```python
from build123d import *

# Parameters (mm, degrees)
F0_W           = 13.375
F0_H           = 2
F1_DEPTH       = 25
F2_R           = 1.75
F3_DEPTH       = 2
F4_W           = 11.3
F4_H           = 33
F5_DEPTH       = 25
F5_DEPTH_BACK  = 11.5
F6_W           = 26
F6_H           = 6.5
F7_DEPTH       = 33
F9_DEPTH       = 33
F11_DEPTH      = 19.75
F11_DEPTH_BACK = 6.25
F12_R          = 1.375
F13_DEPTH      = 4.8
F14_W          = 5.5
F14_H          = 5.5
F15_DEPTH      = 1.5
F16_T1_DEPTH   = 27.75
F16_T3_DEPTH   = 27.75
F16_T5_DEPTH   = 59
F17_T1_DEPTH   = 59.021567647
F17_T3_DEPTH   = 59.021567647
F18_T1_DEPTH   = 6.4746360003
F18_T3_DEPTH   = 20.7323463904
F18_T5_DEPTH   = 52.0573463904
F18_T7_DEPTH   = 15.4323463904
F18_T9_DEPTH   = 14.5286731952
F18_T11_DEPTH  = 6.3286731952
F18_T13_DEPTH  = 6.4746360003
F18_T15_DEPTH  = 1.5286731952
F18_T17_DEPTH  = 7.7786731952
F18_T19_DEPTH  = 7.7786731952
F18_T24_DEPTH  = 4.8857735151
F18_T29_DEPTH  = 10.5573463904
F18_T35_DEPTH  = 4.8857735151
F18_T45_DEPTH  = 14.5286731952
F18_T49_DEPTH  = 7.3573463904
F18_T56_DEPTH  = 8.8073463904
F18_T60_DEPTH  = 2.5573463904
F18_T67_DEPTH  = 4.8857735151
F18_T71_DEPTH  = 10.5573463904
F18_T78_DEPTH  = 10.5573463904
F18_T82_DEPTH  = 4.8857735151
F18_T89_DEPTH  = 2.5573463904
F18_T93_DEPTH  = 8.8073463904


# Not quite as in the source:
# - a fillet or chamfer that OpenCascade refuses, or shapes differently, is made with other operations: its cross-section is extruded or revolved along the edge and cut away or added


with BuildPart() as f1:
    # F0 (on Right) → F1 (new body, symmetric)
    with BuildSketch(Plane.YZ):
        with Locations((6.6875, 1)):
            Rectangle(F0_W, F0_H)
    extrude(amount=F1_DEPTH, both=True)

    # F2 (on face) → F3 (cut, through all)
    with BuildSketch(Plane.XY.offset(2)):
        with Locations((-13, 4)):
            Circle(F2_R)
        with Locations((13, 4)):
            Circle(F2_R)
    extrude(amount=-F3_DEPTH, mode=Mode.SUBTRACT)

    # F4 (on Right) → F5 (join, two sides)
    with BuildSketch(Plane.YZ) as f5_sk:
        with Locations((-5.65, -14.5)):
            Rectangle(F4_W, F4_H)
    extrude(amount=F5_DEPTH)
    extrude(f5_sk.sketch, amount=-F5_DEPTH_BACK)

    # F6 (on face) → F7 (cut, through all)
    with BuildSketch(Plane(origin=(0, 0, -31), x_dir=(1, 0, 0), z_dir=(0, 0, -1))):
        with Locations((6.75, 8.05)):
            Rectangle(F6_W, F6_H)
    extrude(amount=-F7_DEPTH, mode=Mode.SUBTRACT)

    # F8 (on face) → F9 (cut, through all)
    with BuildSketch(Plane(origin=(0, 0, -31), x_dir=(1, 0, 0), z_dir=(0, 0, -1))):
        Polygon((13, 4.8), (0.5, 4.8), (2.5, 2.8), (11, 2.8), align=None)
    extrude(amount=-F9_DEPTH, mode=Mode.SUBTRACT)

    # F10 (on Right) → F11 (cut, two sides)
    with BuildSketch(Plane.YZ) as f11_sk:
        Polygon((-4.8, -31), (-2.8, -31), (-4.8, -19), align=None)
    extrude(amount=F11_DEPTH, mode=Mode.SUBTRACT)
    extrude(f11_sk.sketch, amount=-F11_DEPTH_BACK, mode=Mode.SUBTRACT)

    # F12 (on face) → F13 (cut, through all)
    with BuildSketch(Plane.XZ.offset(4.8)):
        with Locations((-2.5, -16)):
            Circle(F12_R)
        with Locations((16, -16)):
            Circle(F12_R)
    extrude(amount=-F13_DEPTH, mode=Mode.SUBTRACT)

    # F14 (on face) → F15 (cut)
    with BuildSketch(Plane(origin=(0, 0, 0), x_dir=(-1, 0, 0), z_dir=(0, 1, 0))):
        with Locations((-16, -16)):
            Rectangle(F14_W, F14_H)
        with Locations((2.5, -16)):
            Rectangle(F14_W, F14_H)
    extrude(amount=-F15_DEPTH, mode=Mode.SUBTRACT)

    # F16: fillet of radius 4.5 on 3 edges, made by hand

    # F16_s2 → F16_t1 (cut)
    with BuildSketch(Plane.YZ.offset(-22.75)):
        with BuildLine():
            ThreePointArc((-11.3, -26.5), (-9.9819805153, -29.6819805153), (-6.8, -31))
            Line((-6.8, -31), (-11.3, -31))
            Line((-11.3, -31), (-11.3, -26.5))
        make_face()
    extrude(amount=F16_T1_DEPTH, mode=Mode.SUBTRACT)

    # F16_s4 → F16_t3 (cut)
    with BuildSketch(Plane.YZ.offset(8.5)):
        with BuildLine():
            ThreePointArc((-11.3, -26.5), (-9.9819805153, -29.6819805153), (-6.8, -31))
            Line((-6.8, -31), (-11.3, -31))
            Line((-11.3, -31), (-11.3, -26.5))
        make_face()
    extrude(amount=F16_T3_DEPTH, mode=Mode.SUBTRACT)

    # F16_s6 → F16_t5 (cut)
    with BuildSketch(Plane.YZ.offset(-22.75)):
        with BuildLine():
            ThreePointArc((0, -26.5), (-1.3180194847, -29.6819805153), (-4.5, -31))
            Line((-4.5, -31), (0, -31))
            Line((0, -31), (0, -26.5))
        make_face()
    extrude(amount=F16_T5_DEPTH, mode=Mode.SUBTRACT)

    # F17: chamfer of 6 x 10.3923048454 on 2 edges, made by hand

    # F17_s2 → F17_t1 (cut)
    with BuildSketch(Plane.YZ.offset(-38.3857838235)):
        Polygon((-5.3, 2), (-11.3, -8.3923048454), (-11.3, 2), align=None)
    extrude(amount=F17_T1_DEPTH, mode=Mode.SUBTRACT)

    # F17_s4 → F17_t3 (cut)
    with BuildSketch(Plane.YZ.offset(-7.1357838235)):
        Polygon((-5.3, 2), (-11.3, -8.3923048454), (-11.3, 2), align=None)
    extrude(amount=F17_T3_DEPTH, mode=Mode.SUBTRACT)

    # F18: chamfer of 0.4 on 16 edges, made by hand

    # F18_s2 → F18_t1 (cut)
    with BuildSketch(Plane.YZ.offset(19.1376819998)):
        Polygon((-5.4154700538, 1.8), (-5.0690598923, 2), (-5.3, 2), align=None)
    extrude(amount=F18_T1_DEPTH, mode=Mode.SUBTRACT)

    # F18_s4 → F18_t3 (cut)
    with BuildSketch(Plane.XZ.offset(-14.4036731952)):
        Polygon((25, 1.6), (24.6, 2), (25, 2), align=None)
    extrude(amount=F18_T3_DEPTH, mode=Mode.SUBTRACT)

    # F18_s6 → F18_t5 (cut)
    with BuildSketch(Plane.YZ.offset(-26.0286731952)):
        Polygon((13.375, 1.6), (12.975, 2), (13.375, 2), align=None)
    extrude(amount=F18_T5_DEPTH, mode=Mode.SUBTRACT)

    # F18_s8 → F18_t7 (cut)
    with BuildSketch(Plane.XZ.offset(-14.4036731952)):
        Polygon((-25, 1.6), (-24.6, 2), (-25, 2), align=None)
    extrude(amount=F18_T7_DEPTH, mode=Mode.SUBTRACT)

    # F18_s10 → F18_t9 (cut)
    with BuildSketch(Plane.YZ.offset(-26.0286731952)):
        Polygon((0, 1.6), (0.4, 2), (0, 2), align=None)
    extrude(amount=F18_T9_DEPTH, mode=Mode.SUBTRACT)

    # F18_s12 → F18_t11 (cut)
    with BuildSketch(Plane.XZ):
        Polygon((-11.5, 1.6), (-11.1, 2), (-11.5, 2), align=None)
    extrude(amount=F18_T11_DEPTH, mode=Mode.SUBTRACT)

    # F18_s14 → F18_t13 (cut)
    with BuildSketch(Plane.YZ.offset(-12.1123180002)):
        Polygon((-5.4154700538, 1.8), (-5.0690598923, 2), (-5.3, 2), align=None)
    extrude(amount=F18_T13_DEPTH, mode=Mode.SUBTRACT)

    # F18_s16 → F18_t15 (cut)
    with BuildSketch(Plane.XZ.offset(4.8)):
        Polygon((-6.25, 1.6), (-6.65, 2), (-6.25, 2), align=None)
        Polygon((19.75, 1.6), (20.15, 2), (19.75, 2), align=None)
    extrude(amount=F18_T15_DEPTH, mode=Mode.SUBTRACT)

    # F18_s18 → F18_t17 (cut)
    with BuildSketch(Plane.YZ.offset(-6.25)):
        Polygon((-4.8, 1.6), (-4.4, 2), (-4.8, 2), align=None)
    extrude(amount=F18_T17_DEPTH, mode=Mode.SUBTRACT)

    # F18_s20 → F18_t19 (cut)
    with BuildSketch(Plane.YZ.offset(11.9713268048)):
        Polygon((-4.8, 1.6), (-4.4, 2), (-4.8, 2), align=None)
    extrude(amount=F18_T19_DEPTH, mode=Mode.SUBTRACT)


with BuildPart() as f18_tool22:
    # F18_s23 → F18_t24 (new body)
    with BuildSketch(Plane(origin=(-2.8773817919, -2.8773817919, 0), x_dir=(0, 0, 1), z_dir=(0.7071067812, 0.7071067812, 0))):
        Polygon((1.6, 3.7476659403), (2, 3.3476659403), (2, 3.7476659403), align=None)
    extrude(amount=F18_T24_DEPTH)

    split(bisect_by=Plane.XZ.offset(2.8), keep=Keep.TOP)


with BuildPart() as f1_1:
    add(f1.part)

    # F18_t21: cut F18_tool22
    add(f18_tool22.part, mode=Mode.SUBTRACT)


with BuildPart() as f18_tool27:
    # F18_s28 → F18_t29 (new body)
    with BuildSketch(Plane.YZ.offset(1.4713268048)):
        Polygon((-2.8, 1.6), (-2.4, 2), (-2.8, 2), align=None)
    extrude(amount=F18_T29_DEPTH)

    split(bisect_by=Plane(origin=(2.65, -2.65, 0), x_dir=(0, 0, 1), z_dir=(0.7071067812, -0.7071067812, 0)), keep=Keep.TOP)

    split(bisect_by=Plane(origin=(4.1, 4.1, 0), x_dir=(0, 0, 1), z_dir=(-0.7071067812, -0.7071067812, 0)), keep=Keep.TOP)


with BuildPart() as f1_2:
    add(f1_1.part)

    # F18_t26: cut F18_tool27
    add(f18_tool27.part, mode=Mode.SUBTRACT)


with BuildPart() as f18_tool33:
    # F18_s34 → F18_t35 (new body)
    with BuildSketch(Plane(origin=(6.1726182081, -6.1726182081, 0), x_dir=(0, 0, 1), z_dir=(0.7071067812, -0.7071067812, 0))):
        Polygon((1.6, -5.7982756057), (2, -6.1982756057), (2, -5.7982756057), align=None)
    extrude(amount=F18_T35_DEPTH)

    split(bisect_by=Plane.XZ.offset(2.8), keep=Keep.TOP)


with BuildPart() as f1_3:
    add(f1_2.part)

    # F18_t32: cut F18_tool33
    add(f18_tool33.part, mode=Mode.SUBTRACT)

    # F18_s37 → F18_t38 (revolve, cut)
    with BuildSketch(Plane.XZ.offset(-4)):
        Polygon((-11.25, 1.6), (-10.85, 2), (-11.25, 2), align=None)
    revolve(axis=Axis((-13, 4, 2), (0, 0, 1)), mode=Mode.SUBTRACT)

    # F18_s39 → F18_t40 (revolve, cut)
    with BuildSketch(Plane.XZ.offset(-4)):
        Polygon((14.75, 1.6), (15.15, 2), (14.75, 2), align=None)
    revolve(axis=Axis((13, 4, 2), (0, 0, 1)), mode=Mode.SUBTRACT)


with BuildPart() as f18_tool43:
    # F18_s44 → F18_t45 (new body)
    with BuildSketch(Plane.YZ.offset(-10.4713268048)):
        Polygon((0, 1.6), (0.4, 2), (0, 2), align=None)
    extrude(amount=-F18_T45_DEPTH)

    split(bisect_by=Plane.YZ.offset(-11.5), keep=Keep.TOP)


with BuildPart() as f18_tool47:
    # F18_s48 → F18_t49 (new body)
    with BuildSketch(Plane.XZ.offset(-1.0286731952)):
        Polygon((-11.5, 1.6), (-11.1, 2), (-11.5, 2), align=None)
    extrude(amount=F18_T49_DEPTH)

    split(bisect_by=Plane.XZ, keep=Keep.BOTTOM)


with BuildPart() as f18_tool43_1:
    add(f18_tool43.part)

    # F18_t51: intersect F18_tool47
    add(f18_tool47.part, mode=Mode.INTERSECT)


with BuildPart() as f1_4:
    add(f1_3.part)

    # F18_t41: cut F18_tool43
    add(f18_tool43_1.part, mode=Mode.SUBTRACT)


with BuildPart() as f18_tool54:
    # F18_s55 → F18_t56 (new body)
    with BuildSketch(Plane.YZ.offset(-7.2786731952)):
        Polygon((-4.8, 1.6), (-4.4, 2), (-4.8, 2), align=None)
    extrude(amount=F18_T56_DEPTH)

    split(bisect_by=Plane.YZ.offset(-6.25), keep=Keep.BOTTOM)


with BuildPart() as f18_tool58:
    # F18_s59 → F18_t60 (new body)
    with BuildSketch(Plane.XZ.offset(6.3286731952)):
        Polygon((-6.25, 1.6), (-6.65, 2), (-6.25, 2), align=None)
    extrude(amount=-F18_T60_DEPTH)

    split(bisect_by=Plane.XZ.offset(4.8), keep=Keep.BOTTOM)


with BuildPart() as f18_tool54_1:
    add(f18_tool54.part)

    # F18_t62: intersect F18_tool58
    add(f18_tool58.part, mode=Mode.INTERSECT)


with BuildPart() as f1_5:
    add(f1_4.part)

    # F18_t52: cut F18_tool54
    add(f18_tool54_1.part, mode=Mode.SUBTRACT)


with BuildPart() as f18_tool65:
    # F18_s66 → F18_t67 (new body)
    with BuildSketch(Plane(origin=(-2.8773817919, -2.8773817919, 0), x_dir=(0, 0, 1), z_dir=(0.7071067812, 0.7071067812, 0))):
        Polygon((1.6, 3.7476659403), (2, 3.3476659403), (2, 3.7476659403), align=None)
    extrude(amount=F18_T67_DEPTH)

    split(bisect_by=Plane.XZ.offset(2.8), keep=Keep.BOTTOM)


with BuildPart() as f18_tool69:
    # F18_s70 → F18_t71 (new body)
    with BuildSketch(Plane.YZ.offset(1.4713268048)):
        Polygon((-2.8, 1.6), (-2.4, 2), (-2.8, 2), align=None)
    extrude(amount=F18_T71_DEPTH)

    split(bisect_by=Plane(origin=(2.65, -2.65, 0), x_dir=(0, 0, 1), z_dir=(-0.7071067812, 0.7071067812, 0)), keep=Keep.TOP)


with BuildPart() as f18_tool65_1:
    add(f18_tool65.part)

    # F18_t73: intersect F18_tool69
    add(f18_tool69.part, mode=Mode.INTERSECT)


with BuildPart() as f1_6:
    add(f1_5.part)

    # F18_t63: cut F18_tool65
    add(f18_tool65_1.part, mode=Mode.SUBTRACT)


with BuildPart() as f18_tool76:
    # F18_s77 → F18_t78 (new body)
    with BuildSketch(Plane.YZ.offset(1.4713268048)):
        Polygon((-2.8, 1.6), (-2.4, 2), (-2.8, 2), align=None)
    extrude(amount=F18_T78_DEPTH)

    split(bisect_by=Plane(origin=(4.1, 4.1, 0), x_dir=(0, 0, 1), z_dir=(0.7071067812, 0.7071067812, 0)), keep=Keep.TOP)


with BuildPart() as f18_tool80:
    # F18_s81 → F18_t82 (new body)
    with BuildSketch(Plane(origin=(6.1726182081, -6.1726182081, 0), x_dir=(0, 0, 1), z_dir=(0.7071067812, -0.7071067812, 0))):
        Polygon((1.6, -5.7982756057), (2, -6.1982756057), (2, -5.7982756057), align=None)
    extrude(amount=F18_T82_DEPTH)

    split(bisect_by=Plane.XZ.offset(2.8), keep=Keep.BOTTOM)


with BuildPart() as f18_tool76_1:
    add(f18_tool76.part)

    # F18_t84: intersect F18_tool80
    add(f18_tool80.part, mode=Mode.INTERSECT)


with BuildPart() as f1_7:
    add(f1_6.part)

    # F18_t74: cut F18_tool76
    add(f18_tool76_1.part, mode=Mode.SUBTRACT)


with BuildPart() as f18_tool87:
    # F18_s88 → F18_t89 (new body)
    with BuildSketch(Plane.XZ.offset(3.7713268048)):
        Polygon((19.75, 1.6), (20.15, 2), (19.75, 2), align=None)
    extrude(amount=F18_T89_DEPTH)

    split(bisect_by=Plane.XZ.offset(4.8), keep=Keep.BOTTOM)


with BuildPart() as f18_tool91:
    # F18_s92 → F18_t93 (new body)
    with BuildSketch(Plane.YZ.offset(11.9713268048)):
        Polygon((-4.8, 1.6), (-4.4, 2), (-4.8, 2), align=None)
    extrude(amount=F18_T93_DEPTH)

    split(bisect_by=Plane.YZ.offset(19.75), keep=Keep.TOP)


with BuildPart() as f18_tool87_1:
    add(f18_tool87.part)

    # F18_t95: intersect F18_tool91
    add(f18_tool91.part, mode=Mode.INTERSECT)


with BuildPart() as f1_8:
    add(f1_7.part)

    # F18_t85: cut F18_tool87
    add(f18_tool87_1.part, mode=Mode.SUBTRACT)


solid = f1_8.part
```
Here's how the part is built. I have some questions about the finished solid (model axes, mm). A direction names the side the tool comes from. Coordinates: 2 decimals unless noted, no trailing zeros. Write each loop counter-clockwise with the first axis right and the second up, starting at its lowest first coordinate (ties: lowest second). Pieces come first, ordered by that corner, then holes. Notation, with made-up numbers: (47.5, 49.25) -> (55.5, 49.25) arc R25 cw to (55.5, 81.25) -> close; hole circle Ø2 at (38.5, 85.5). An arc over 180 degrees is marked (long way). Use a Markdown table: item, result. Add a question column.
(1) If we section it at D-D, the plane x = 6.5: Write out the boundary of the cut face in (y, z) (3 decimals), and give its area (3 significant figures).
(2) I'm going to push flat-ended pins straight in: P1, Ø4.5, axis at x = 16, z = -15, coming from the +Y side; P2, Ø1.6, axis at y = -1, z = -17, coming from the -X side; P3, Ø12, axis at x = 8, z = -20.5, coming from the -Y side. Where does each tip first touch, or does it pass through?
(3) If we section it at B-B, the plane y = 4: Write out the boundary of the cut face in (x, z), and give its area (3 significant figures).
(4) If we section it at C-C, the plane z = -16: Write out the boundary of the cut face in (x, y) (3 decimals).
(5) If we section it at A-A, the plane x = -13: Write out the boundary of the cut face in (y, z) (3 decimals).
(6) For faces 1 (the flat face through (-2, -1, -13.25)), 2 (the flat face through (7, 0, -13)), 3 (the flat face through (1.5, -3.8, -11.2)), 4 (the flat face through (16.31, -3.81, -24.93)), which set-ups out of +Z, -Z, +X, -X, +Y, -Y let a thin tool reach every point of the face, with its end or its side?
(7) Please list where these lines run through material, in increasing order: line 1 (Y direction, x = 13, z = 1.25) (3 decimals); line 2 (X direction, y = -8.75, z = -9); line 3 (Y direction, x = -13, z = 1.35) (3 decimals).
Outcome:
| question | item | result |
|---|---|---|
| 1 | outline | (-2.8, -30.667) arc R4.5 ccw to (0, -26.5) -> (0, 0) -> (13.375, 0) -> (13.375, 1.6) -> (12.975, 2) -> (-2.4, 2) -> (-2.8, 1.6) -> close |
| 1 | area | 115 mm^2 |
| 2 | P1 | stops at y = 0 |
| 2 | P2 | stops at x = -11.5 |
| 2 | P3 | stops at y = -4.8 |
| 3 | outline | (-25, 0) -> (-14.75, 0) -> (-14.75, 1.6) -> (-15.15, 2) -> (-24.6, 2) -> (-25, 1.6) -> close; (-11.25, 0) -> (11.25, 0) -> (11.25, 1.6) -> (10.85, 2) -> (-10.85, 2) -> (-11.25, 1.6) -> close; (14.75, 0) -> (25, 0) -> (25, 1.6) -> (24.6, 2) -> (15.15, 2) -> (14.75, 1.6) -> close |
| 3 | area | 85.5 mm^2 |
| 4 | outline | (-11.5, -11.3) -> (-6.25, -11.3) -> (-6.25, -4.8) -> (-3.875, -4.8) -> (-3.875, -1.5) -> (-5.25, -1.5) -> (-5.25, 0) -> (-11.5, 0) -> close; (-1.125, -4.8) -> (0.5, -4.8) -> (2.5, -2.8) -> (11, -2.8) -> (13, -4.8) -> (14.625, -4.8) -> (14.625, -1.5) -> (13.25, -1.5) -> (13.25, 0) -> (0.25, 0) -> (0.25, -1.5) -> (-1.125, -1.5) -> close; (17.375, -4.8) -> (19.75, -4.8) -> (19.75, -11.3) -> (25, -11.3) -> (25, 0) -> (18.75, 0) -> (18.75, -1.5) -> (17.375, -1.5) -> close |
| 5 | outline | (0, 0) -> (2.25, 0) -> (2.25, 1.6) -> (1.85, 2) -> (0.4, 2) -> (0, 1.6) -> close; (5.75, 0) -> (13.375, 0) -> (13.375, 1.6) -> (12.975, 2) -> (6.15, 2) -> (5.75, 1.6) -> close |
| 6 | face 1 | +Y |
| 6 | face 2 | -Z, +X, -X, +Y |
| 6 | face 3 | +Z, -Z, -Y |
| 6 | face 4 | -Z, -Y |
| 7 | line 1 | y = -4.8 to 2.25, 5.75 to 13.375 |
| 7 | line 2 | x = -11.5 to -6.25, 19.75 to 25 |
| 7 | line 3 | y = 0 to 2.25, 5.75 to 13.375 |
